Input: part model. Units: mm. Frame: model coordinates. Round coordinates to 2 decimals unless told otherwise and drop trailing zeros. Loops run counter-clockwise (first coordinate to the right, second up) from the corner with the lowest first, then second, coordinate; pieces in that order, holes last. Notation, with made-up numbers: (-16, 31) -> (1, 31) arc R27 cw to (1, 57) -> close; hole circle Ø8 at (-21.75, -14). An arc over 180 degrees is marked (long way). Answer as a JSON object with one key per item and string values.
```python
from build123d import *


with BuildPart() as part:
    # Sketch1 → Revolve1 (revolve)
    with BuildSketch(Plane.XY, mode=Mode.PRIVATE) as revolve1_sk:
        with BuildLine():
            Line((1.5, 0), (2.963907916, 0))
            ThreePointArc((2.963907916, 0), (3.116511912, -0.070725021), (3.1611867, -0.232879797))
            Line((3.1611867, -0.232879797), (2.727853367, -2.832879797))
            ThreePointArc((2.727853367, -2.832879797), (2.659849562, -2.952603996), (2.530574582, -3))
            Line((2.530574582, -3), (2.2, -3))
            Line((2.2, -3), (2.2, -1.32133537))
            Line((2.2, -1.32133537), (1.7, -1.32133537))
            ThreePointArc((1.7, -1.32133537), (1.558578644, -1.262756726), (1.5, -1.12133537))
            Line((1.5, -1.12133537), (1.5, 0))
        make_face()
    revolve(revolve1_sk.sketch.rotate(Axis((0, 1.955447774, 0), (0, -1, 0)), 90), axis=Axis((0, 1.955447774, 0), (0, -1, 0)))


solid = part.part
```
1) Contact query for flat-ended pins moving along their axis: P1, Ø1, axis at y = -0.5, z = 1.5, coming from the +X side; P2, Ø3.5, axis at x = 0, z = 0, coming from the -Y side. Output: stop coordinate, or through.
Output:
{"P1": "stops at x = 2.97", "P2": "stops at y = -1.32"}
2) Section B-B, the plane x = 0. Output: boundary loops of the cut face in (y, z).
Output:
{"outline": "(-3, -2.53) arc R0.2 ccw to (-2.83, -2.73) -> (-0.23, -3.16) arc R0.2 ccw to (0, -2.96) -> (0, -1.5) -> (-1.12, -1.5) arc R0.2 ccw to (-1.32, -1.7) -> (-1.32, -2.2) -> (-3, -2.2) -> close; (-3, 2.2) -> (-1.32, 2.2) -> (-1.32, 1.7) arc R0.2 ccw to (-1.12, 1.5) -> (0, 1.5) -> (0, 2.96) arc R0.2 ccw to (-0.23, 3.16) -> (-2.83, 2.73) arc R0.2 ccw to (-3, 2.53) -> close"}
3) Section C-C, the plane y = -1.8. Output: boundary loops of the cut face in (x, z), plus the area to 3 significant figures.
Output:
{"outline": "circle Ø5.8 at (0, 0); hole circle Ø4.4 at (0, 0)", "area": "11.2 mm^2"}
4) Section A-A, the plane z = 0. Output: boundary loops of the cut face in (x, y).
Output:
{"outline": "(-3.16, -0.23) -> (-2.73, -2.83) arc R0.2 ccw to (-2.53, -3) -> (-2.2, -3) -> (-2.2, -1.32) -> (-1.7, -1.32) arc R0.2 ccw to (-1.5, -1.12) -> (-1.5, 0) -> (-2.96, 0) arc R0.2 ccw to start; (1.5, -1.12) arc R0.2 ccw to (1.7, -1.32) -> (2.2, -1.32) -> (2.2, -3) -> (2.53, -3) arc R0.2 ccw to (2.73, -2.83) -> (3.16, -0.23) arc R0.2 ccw to (2.96, 0) -> (1.5, 0) -> close"}
5) Section D-D, the plane y = -2.5. Output: boundary loops of the cut face in (x, z), plus the area to 3 significant figures.
Output:
{"outline": "circle Ø5.57 at (0, 0); hole circle Ø4.4 at (0, 0)", "area": "9.13 mm^2"}
6) Ray query, probe 1 along Z at (x, y) = (-1, -1.4); probe 2 along X at (y, z) = (-2.1, 0); probe 3 along Z at (x, y) = (-0.25, -0.8). Return the intervals inside material, ascending.
Output:
{"probe 1": "z = -2.79 to -1.96, 1.96 to 2.79", "probe 2": "x = -2.85 to -2.2, 2.2 to 2.85", "probe 3": "z = -3.06 to -1.48, 1.48 to 3.06"}
7) Draft query along X for faces 1 (the face through (0, -1.321, -2)), 2 (the face through (-2.18, -2.15, -0.29)), 3 (the face through (-0.855, -2.129, 2.714)), 4 (the face through (1.3, 0, -1.3)). Return one class per face: +X half, -X half, draft (parallel to the pull), parting line (faces both ways), or undercut.
Output:
{"face 1": "undercut", "face 2": "undercut", "face 3": "parting line", "face 4": "draft"}
